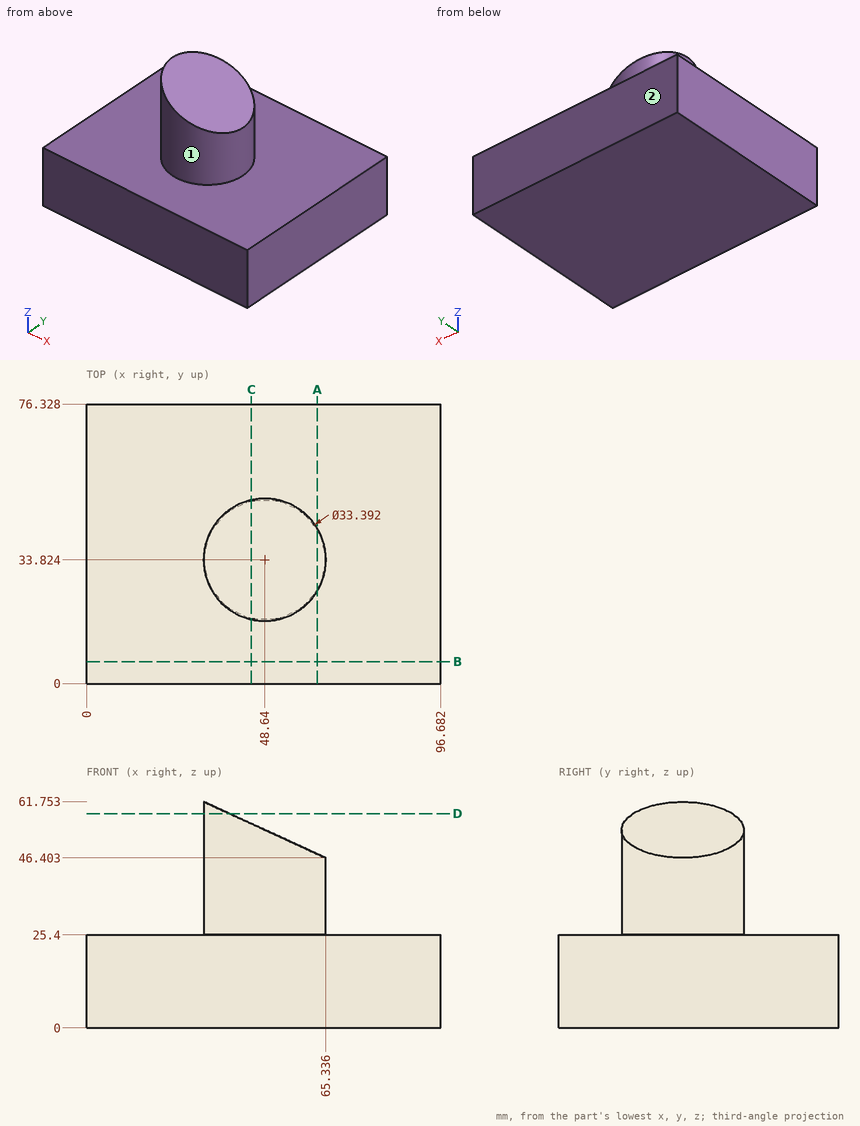
Source: three-view drawing plus pictorial views. Frame: mm from the lowest corner of the part. A direction names the side the tool comes from. Coordinates: 2 decimals unless noted, no trailing zeros. Loops run counter-clockwise (first coordinate to the right, second up) from the corner with the lowest first, then second, coordinate; pieces in that order, holes last. Notation, with made-up numbers: (0, 55.25) -> (57, 55.25) arc R15 ccw to (57, 79.25) -> close; hole circle Ø9 at (47, 23). An arc over 180 degrees is marked (long way). One line per item, written item: value.
(1) Ray query, line 1 along Z through (x, y) = (45.5, 10.5); line 2 along Y through (x, z) = (49.5, 52); line 3 along Y through (x, z) = (48, 39). Return the intervals inside material, ascending.
Answer below:
line 1: z = 0 to 25.4
line 2: y = 17.15 to 50.5
line 3: y = 17.14 to 50.51
(2) Cut plane A-A (x = 63). Output: boundary loops of the cut face in (y, z) (1 decimal), then the cut area to 4 significant figures.
Answer below:
outline: (0, 0) -> (76.3, 0) -> (76.3, 25.4) -> (42.3, 25.4) -> (42.3, 47.5) -> (25.3, 47.5) -> (25.3, 25.4) -> (0, 25.4) -> close
area: 2,315 mm2
(3) Set-up query: the marked faces 1 and 2. Return all of +Z, -Z, +X, -X, +Y, -Y with unobstructed straight access to the full face (end or side cutting, diameter ignored); none if empty.
Answer below:
face 1: +Z
face 2: +Z, -Z, +X, -X, +Y
(4) Cut plane B-B (y = 6). Output: boundary loops of the cut face in (x, z), then the cut area to 3 significant figures.
Answer below:
outline: (0, 0) -> (96.68, 0) -> (96.68, 25.4) -> (0, 25.4) -> close
area: 2,460 mm2
(5) Cut plane D-D (z = 58.5). Output: boundary loops of the cut face in (x, y) (1 decimal), then the cut area to 3 significant figures.
Answer below:
outline: (39, 20.2) -> (39, 47.5) arc R16.7 ccw to start
area: 135 mm2
(6) Cut plane C-C (x = 45). Output: boundary loops of the cut face in (y, z).
Answer below:
outline: (0, 0) -> (76.33, 0) -> (76.33, 25.4) -> (50.12, 25.4) -> (50.12, 55.75) -> (17.53, 55.75) -> (17.53, 25.4) -> (0, 25.4) -> close
(7) Pin query (flat end, axial travel): pin 1 Ø2 at (x, y) = (45, 35) entering from +Z; pin 2 Ø5 at (x, y) = (46.5, 10) entering from +Z; pin 3 Ø1 at (x, y) = (41.5, 37) entering from +Z. Return the tip coordinate at first contact, or that it passes through.
Answer below:
pin 1: stops at z = 56.21
pin 2: stops at z = 25.4
pin 3: stops at z = 57.59
